from build123d import *

# Parameters (mm, degrees)
SKETCH1_R = 63.5


with BuildPart() as part:
    # Sweep1: sweep along a path in Sketch2
    with BuildLine(Plane(origin=(0, 0, 0), x_dir=(0, 0, -1), z_dir=(1, 0, 0))) as sweep1_path:
        Line((0, 0), (177.8, 0))
        ThreePointArc((177.8, 0), (304.8, -127), (177.8, -254))
        Line((177.8, -254), (-203.2, -254))
        ThreePointArc((-203.2, -254), (-330.2, -127), (-203.2, 0))
        Line((-203.2, 0), (-2.54, 0))
    # Sketch1 → Sweep1 (sweep)
    with BuildSketch(Plane.XY):
        Circle(SKETCH1_R)
    sweep(path=sweep1_path.line)


solid = part.part
Here's how the part is built. I have some questions about the finished solid (model axes, mm). A direction names the side the tool comes from. Round coordinates to 2 decimals unless told otherwise and drop trailing zeros. Loops run counter-clockwise (first coordinate to the right, second up) from the corner with the lowest first, then second, coordinate; pieces in that order, holes last.
1. For P1, Ø10, axis at x = 37, y = -56, coming from the -Z side; P2, Ø1, axis at y = -273, z = 43, coming from the -X side; P3, Ø10, axis at x = -28.5, y = -228.5, coming from the +Z side, each with a flat end and sliding along its axis, tell me the tip position at first contact or that it passes through.
Answer list:
P1: stops at z = -345.83
P2: stops at x = -60.75
P3: stops at z = 360.61
2. If I drill on line 1 along X through (y, z) = (-2, -211); line 2 along Z through (x, y) = (28, -9.5); line 3 along Z through (x, y) = (21, -146), over which ranges is the centre line in solid material (lowest first)?
Answer list:
line 1: x = -63.46 to 63.46
line 2: z = -319.39 to 0, 2.54 to 344.79
line 3: z = -363.76 to -242.13, 267.53 to 389.16
3. Which directions (+Z, -Z, +X, -X, +Y, -Y) give clear straight access to the entire face, cutting with the end or side of a thin tool? Please do faces 1 (the face through (-1, 1, 2.54)), 2 (the face through (-13.77, 61.99, 101.47)).
Answer list:
face 1: +X, -X, +Y
face 2: none
4. If we section it at B-B on z = -144: Write out the boundary of the cut face in (x, y), plus the area to 3 significant figures.
Answer list:
outline: circle Ø127 at (0, -254); circle Ø127 at (0, 0)
area: 25,300 mm2
5. If we section it at A-A on x = 0: Write out the boundary of the cut face in (y, z), plus the area to 3 significant figures.
Answer list:
outline: (-317.5, -177.8) arc R190.5 ccw to (63.5, -177.8) - (63.5, 0) - (-63.5, 0) - (-63.5, -177.8) arc R63.5 cw to (-190.5, -177.8) - (-190.5, 203.2) arc R63.5 cw to (-63.5, 203.2) - (-63.5, 2.54) - (63.5, 2.54) - (63.5, 203.2) arc R190.5 ccw to (-317.5, 203.2) - close
area: 198,000 mm2
6. If we section it at C-C on x = 49: Write out the boundary of the cut face in (y, z), plus the area to 3 significant figures.
Answer list:
outline: (-294.39, -177.8) arc R167.39 ccw to (40.39, -177.8) - (40.39, 0) - (-40.39, 0) - (-40.39, -177.8) arc R86.61 cw to (-213.61, -177.8) - (-213.61, 203.2) arc R86.61 cw to (-40.39, 203.2) - (-40.39, 2.54) - (40.39, 2.54) - (40.39, 203.2) arc R167.39 ccw to (-294.39, 203.2) - close
area: 126,000 mm2
